```python
from build123d import *

# Parameters (mm, degrees)
SKETCH1_W           = 96
SKETCH1_H           = 64
BOSS_EXTRUDE1_DEPTH = 16
CUT_EXTRUDE1_DEPTH  = 16
BOSS_EXTRUDE2_DEPTH = 16
CHAMFER1_SIZE       = 20
CHAMFER1_SIZE2      = 30
SKETCH5_W           = 40
SKETCH5_H           = 28
BOSS_EXTRUDE3_DEPTH = 42
SKETCH6_R           = 12
CUT_EXTRUDE2_DEPTH  = 42
BOSS_EXTRUDE4_DEPTH = 12


with BuildPart() as part:
    # Sketch1 → Boss-Extrude1 (new body)
    with BuildSketch(Plane(origin=(0, 0, 0), x_dir=(1, 0, 0), z_dir=(0, 1, 0))):
        with Locations((-25.220534577, -0.638984057)):
            Rectangle(SKETCH1_W, SKETCH1_H)
    extrude(amount=BOSS_EXTRUDE1_DEPTH)

    # Sketch2 → Cut-Extrude1 (cut)
    with BuildSketch(Plane(origin=(0, 16, 0), x_dir=(1, 0, 0), z_dir=(0, 1, 0))):
        with BuildLine():
            Line((22.779465423, -8.638984057), (2.779465423, -8.638984057))
            ThreePointArc((2.779465423, -8.638984057), (-5.220534577, -0.638984057), (2.779465423, 7.361015943))
            Line((2.779465423, 7.361015943), (22.779465423, 7.361015943))
            ThreePointArc((22.779465423, 7.361015943), (30.779465423, -0.638984057), (22.779465423, -8.638984057))
        make_face()
    extrude(amount=-CUT_EXTRUDE1_DEPTH, mode=Mode.SUBTRACT)

    # Sketch3 → Boss-Extrude2 (add)
    with BuildSketch(Plane.ZY.offset(73.220534577)):
        Polygon((32.638984057, 16), (32.638984057, 80), (-31.362039682, 80), (-31.361015943, 16), align=None)
    extrude(amount=-BOSS_EXTRUDE2_DEPTH)

    # Chamfer1
    chamfer1_edges = [part.edges().sort_by_distance(p)[0] for p in [
        (-65.220534577, 80, 32.638984057),
    ]]
    chamfer1_side = [part.faces().sort_by_distance(p)[0] for p in [
        (-65.220534577, 80, 0.638472187),
    ]]
    chamfer(chamfer1_edges, length=CHAMFER1_SIZE, length2=CHAMFER1_SIZE2, reference=chamfer1_side[0])

    # Sketch5 → Boss-Extrude3 (add)
    with BuildSketch(Plane(origin=(0, 0, -31.361015943), x_dir=(-1, 0, 0), z_dir=(0, 0, -1))):
        with Locations((37.220534577, 30)):
            Rectangle(SKETCH5_W, SKETCH5_H)
    extrude(amount=-BOSS_EXTRUDE3_DEPTH)

    # Sketch6 → Cut-Extrude2 (cut)
    with BuildSketch(Plane.XY.offset(10.638984057)):
        with Locations((-37.220534577, 44)):
            Circle(SKETCH6_R)
    extrude(amount=-CUT_EXTRUDE2_DEPTH, mode=Mode.SUBTRACT)

    # Sketch7 → Boss-Extrude4 (add)
    with BuildSketch(Plane(origin=(0, 0, -31.361015943), x_dir=(-1, 0, 0), z_dir=(0, 0, -1))):
        Polygon((-22.779465423, 16), (17.220534577, 44), (17.220534577, 16), align=None)
    extrude(amount=-BOSS_EXTRUDE4_DEPTH)


solid = part.part
```
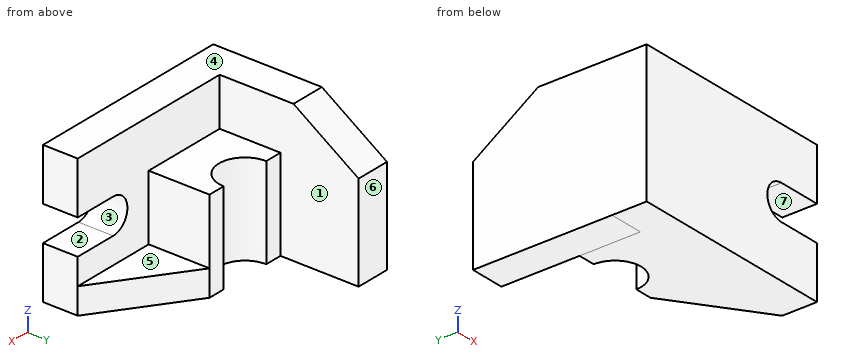
Part model, mm, in its own coordinate system. Face numbers are marked on the shaded views. A direction names the side the tool comes from. Round coordinates to 2 decimals unless told otherwise and drop trailing zeros. Loops run counter-clockwise (first coordinate to the right, second up) from the corner with the lowest first, then second, coordinate; pieces in that order, holes last.
Item 1: 3-axis set-ups, long thin cutter, end or side, ignore diameter. For the marked faces 5, 6 and 7: which of +Z, -Z, +X, -X, +Y, -Y reach the whole face in a straight line?
Item 2: Cut at D-D, the plane y = 63.5. Give the cut face in (x, z).
Item 3: Cut at C-C, the plane z = -10.5. Give the cut face in (x, y), then the cut area to 3 significant figures.
Item 4: Drill centre lines: line 1 (Z direction, x = -16, y = 9); line 2 (Y direction, x = -4, z = -17); line 3 (X direction, y = 27.5, z = -15.5). Where is each one in solid material? Low to high.
Item 5: Mould opens along Z. For the marked faces 1, 2, 3 and 4 say: +Z half, -Z half, draft (parallel to the pull), parting line (faces both ways), or undercut.
Item 6: Cut at B-B, the plane x = -66.5. Give the cut face in (y, z), then the cut area to 3 significant figures.
Item 7: Cut at A-A, the plane x = 13.5. Give the cut face in (y, z), then the cut area to 3 significant figures.
Item 8: Drop flat-ended pins along their axis: P1, Ø2.5, axis at x = -22, z = -9, coming from the +Y side; P2, Ø1, axis at y = 39.5, z = -10, coming from the +X side; P3, Ø15.5, axis at x = -24.5, z = 19, coming from the +Y side. Give the stop position or say it passes through.
A:
1. face 5: +Z, +X, +Y
1. face 6: +Z, -Z, +X, -X, +Y
1. face 7: +X, +Y, -Y
2. outline: (-73.22, -31.36) - (-57.22, -31.36) - (-57.22, 23.64) - (-73.22, 23.64) - close
3. outline: (-73.22, 0) - (22.78, 0) - (22.78, 16) - (-17.22, 16) - (-17.22, 44) - (-25.22, 44) arc R12 cw to (-49.22, 44) - (-57.22, 44) - (-57.22, 80) - (-73.22, 80) - close
3. area: 3,450 mm2
4. line 1: z = -31.36 to 32.64
4. line 2: y = 0 to 16
4. line 3: x = -73.22 to -17.22
5. face 1: draft
5. face 2: undercut
5. face 3: undercut
5. face 4: +Z half
6. outline: (0, -31.36) - (16, -31.36) - (80, -31.36) - (80, 12.64) - (50, 32.64) - (0, 32.64) - close
6. area: 4,820 mm2
7. outline: (0, -31.36) - (22.5, -31.36) - (22.5, -19.36) - (16, -19.36) - (16, -7.36) - (0, -7.36) - close; (0, 8.64) - (16, 8.64) - (16, 32.64) - (0, 32.64) - close
7. area: 846 mm2
8. P1: stops at y = 44
8. P2: stops at x = -17.22
8. P3: stops at y = 16
